The listing builds one solid part. Answer for the finished solid, in the listing's coordinates (mm). A direction names the side the tool comes from. Round coordinates to 2 decimals unless told otherwise and drop trailing zeros. Write each loop counter-clockwise with the first axis right and the second up, starting at its lowest first coordinate (ties: lowest second). Pieces come first, ordered by that corner, then holes. Notation, with made-up numbers: (67, 74) - (100, 74) arc R9 ccw to (100, 85) - close; hole circle Ø3 at (-30.5, 35.5). An arc over 180 degrees is marked (long way). Return JSON: item names as keys, results as strings. Group by question number.
from build123d import *

# Parameters (mm, degrees)
SKETCH_1_R               = 3.5
EXTRUDE_2_DEPTH          = 34
CUT_EXTRUDE_1_DEPTH      = 42.388404173
CUT_EXTRUDE_1_DEPTH_BACK = 42.388404173
SKETCH_3_W               = 8
SKETCH_3_H               = 13
SKETCH_4_R               = 5.05
CUT_EXTRUDE_3_DEPTH      = 10


with BuildPart() as part:
    # 草图1 → 凸台-拉伸2 (new body)
    with BuildSketch(Plane.XY):
        with BuildLine():
            Line((7, 5), (7, -5))
            Line((7, -5), (-7, -5))
            Line((-7, -5), (-7, 5))
            Line((-7, 5), (-6, 13))
            ThreePointArc((-6, 13), (0, 19), (6, 13))
            Line((6, 13), (7, 5))
        make_face()
        with Locations((0, 13)):
            Circle(SKETCH_1_R, mode=Mode.SUBTRACT)
    extrude(amount=EXTRUDE_2_DEPTH)

    # 草图3 → 切除-拉伸1 (cut, two sides: drawn at the far end of the back side and taken through both)
    with BuildSketch(Plane(origin=(7, 0, 0), x_dir=(0, 0, -1), z_dir=(1, 0, 0)).offset(-CUT_EXTRUDE_1_DEPTH_BACK)):
        with Locations((-23.713626646, 12.5)):
            Rectangle(SKETCH_3_W, SKETCH_3_H)
        Polygon((-6.286373354, 19), (-13.713626646, 19), (-14.286373354, 19), (-14.286373354, 6), (-6.286373354, 6), align=None)
    extrude(amount=CUT_EXTRUDE_1_DEPTH + CUT_EXTRUDE_1_DEPTH_BACK, mode=Mode.SUBTRACT)

    # 草图4 → 切除-拉伸3 (cut)
    with BuildSketch(Plane.XZ.offset(5)):
        with Locations((-0.001873454, 27)):
            Circle(SKETCH_4_R)
        with Locations((-0.001873454, 7)):
            Circle(SKETCH_4_R)
    extrude(amount=-CUT_EXTRUDE_3_DEPTH, mode=Mode.SUBTRACT)


solid = part.part
(1) Find section B-B (z = 15). Write down the section's boundary in (x, y), plus the area to 3 significant figures.
(2) Flat-ended cylindrical pins translate along their axes: pin 1 (5.5 mm diameter, centred on x = 0, y = 13, fed in from +Z); pin 2 (1.5 mm diameter, centred on x = -2.5, z = 29.5, fed in from -Y). Find the tip coordinate at first contact, or state that the pin passes through.
(3) Find section A-A (x = 0). State how many separate pieces and enclosed holes the cut face has, plus the area to 3 significant figures.
(4) Determine the mould class of faces 4 (the flat face through (1.4, 9.5, 19.714)), 5 (the flat face through (7, 0, 17)), 6 (the flat face through (0, 5, 34)) for opening direction Z: +Z half, -Z half, draft (parallel to the pull), parting line (faces both ways), or undercut.
(5) Consider line 1 (Z direction, x = 6, y = 12.5); line 2 (X direction, y = 13, z = 3); line 3 (Z direction, x = 3.25, y = -1.25). Determine where each line is inside the solid, lowest interval first.
(6) Find section C-C (y = -0.25). Write down the section's boundary in (x, z), plus the area to 3 significant figures.
(7) Find section D-D (y = 6.5). Write down the section's boundary in (x, z), plus the area to 3 significant figures.
(8) For faces 1 (the cylindrical face through (-0.759, 9.583, 3.099)), 2 (the flat face through (0, 5, 27)), 3 (the flat face through (-1.6, 9.7, 14.286)), determine the directions among +Z, -Z, +X, -X, +Y, -Y from which every point of the face is accessible in a straight line to the end or side of a thin tool.
Check sheet entries:
{
 "1": {"outline": "(-7, -5) - (7, -5) - (7, 5) - (6, 13) arc R6 ccw to (-6, 13) - (-7, 5) - close; hole circle Ø7 at (0, 13)", "area": "262 mm^2"},
 "2": {"pin 1": "passes through", "pin 2": "stops at y = 5"},
 "3": {"separate pieces": "4", "enclosed holes": "0", "area": "280 mm^2"},
 "4": {"face 4": "undercut", "face 5": "draft", "face 6": "+Z half"},
 "5": {"line 1": "z = 0 to 6.29, 14.29 to 19.71, 27.71 to 34", "line 2": "x = -6 to -3.5, 3.5 to 6", "line 3": "z = 0 to 3.14, 10.86 to 23.14, 30.86 to 34"},
 "6": {"outline": "(-7, 0) - (7, 0) - (7, 34) - (-7, 34) - close; hole circle Ø10.1 at (0, 7); hole circle Ø10.1 at (0, 27)", "area": "316 mm^2"},
 "7": {"outline": "(-6.81, 0) - (6.81, 0) - (6.81, 6.29) - (-6.81, 6.29) - close; (-6.81, 14.29) - (6.81, 14.29) - (6.81, 19.71) - (-6.81, 19.71) - close; (-6.81, 27.71) - (6.81, 27.71) - (6.81, 34) - (-6.81, 34) - close", "area": "245 mm^2"},
 "8": {"face 1": "+Z, -Z", "face 2": "-Y", "face 3": "+X, -X, +Y"}
}
